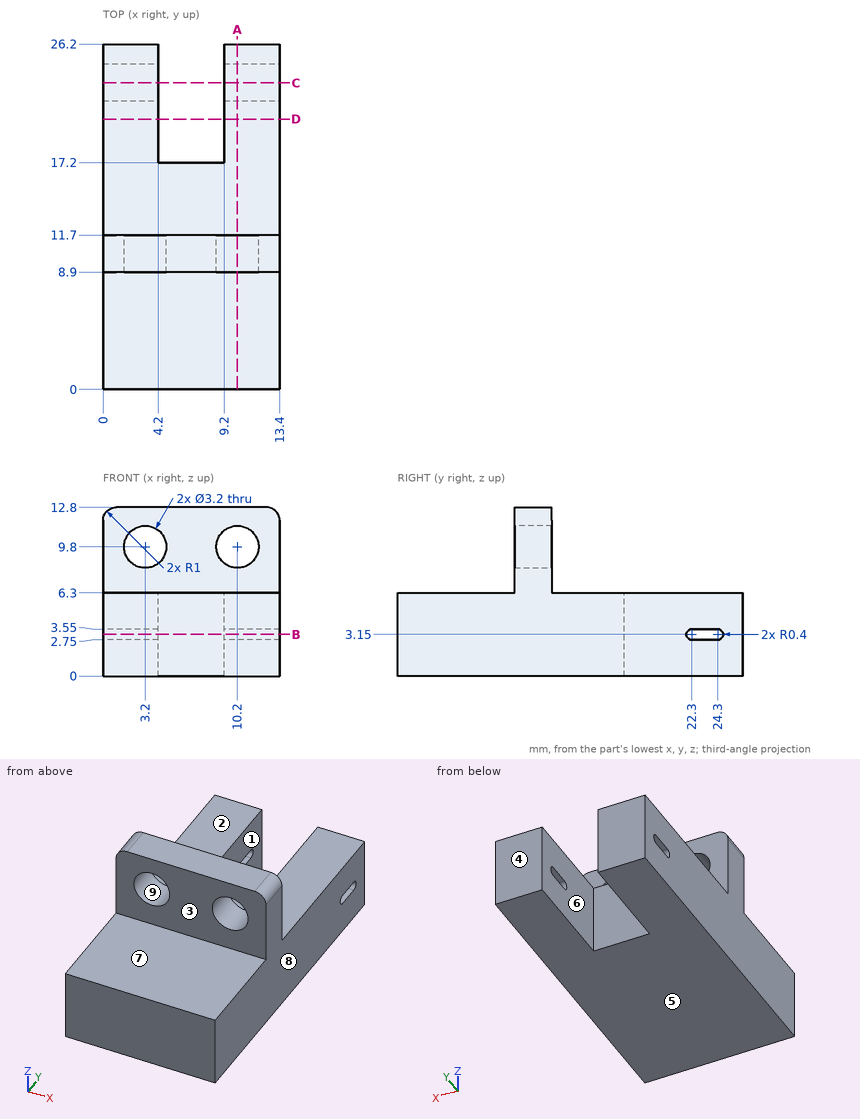
Job drawing, mm, ordinate dimensions from the low corner. One solid piece. A direction names the side the tool comes from. Give positions to 0.01 mm unless a question says otherwise; leave off trailing zeros. Write each loop counter-clockwise with the first axis right and the second up, starting at its lowest first coordinate (ties: lowest second). Pieces come first, ordered by that corner, then holes. Notation, with made-up numbers: M 15.5,47.25 L 47.5,47.25 A11 ccw 47.5,61.25 Z; hole C -11.75,70 d10. An arc over 180 degrees is marked long. Put each result on its own line as item: value. Start each with the question number.
(1) Band-saw the part on C-C, the plane y = 23.25. Write the cut outline in (x, z).
(2) Mould opens along X. For the marked faces 6, 7, 8 and 9 say: +X half, -X half, draft (parallel to the pull), parting line (faces both ways), or undercut.
(3) Which spindle directions (+Z, -Z, +X, -X, +Y, -Y) get a long thin tool onto all of the face, cutting with end or side? Do the marked faces 1, 2, 3, 4 and 5. Say none if no direction does.
(4) Flat gauge pins, fed straight in: pin 1 Ø7 at (x, z) = (5, 10) entering from +Y; pin 2 Ø1.5 at (x, z) = (6, 8) entering from -Y; pin 3 Ø0.6 at (x, y) = (1.5, 23.5) entering from +Z; pin 4 Ø1.9 at (x, z) = (3.2, 9.8) entering from +Y. Where does each tip first touch, or does it go through?
(5) Band-saw the part on A-A, the plane x = 10.2. Write the cut outline in (y, z).
(6) Band-saw the part on B-B, the plane z = 3.15. Write the cut outline in (x, y).
(7) Band-saw the part on D-D, the plane y = 20.5. Write the cut outline in (x, z), and give its area (3 significant figures).
(8) Probe L1, parallel to X at y = 11.1, z = 9.8; L2, parallel to Z at x = 12.5, y = 23.5; L3, parallel to Y at x = 8.25, z = 11.5. List the from-to ranges inside material, lowest first.
Response values:
1. outline: M 0,0 L 4.2,0 L 4.2,2.75 L 0,2.75 Z; M 0,3.55 L 4.2,3.55 L 4.2,6.3 L 0,6.3 Z; M 9.2,0 L 13.4,0 L 13.4,2.75 L 9.2,2.75 Z; M 9.2,3.55 L 13.4,3.55 L 13.4,6.3 L 9.2,6.3 Z
2. face 6: undercut
2. face 7: draft
2. face 8: +X half
2. face 9: undercut
3. face 1: +Z, -Z, +Y
3. face 2: +Z, +X, -X, +Y
3. face 3: +Z, +X, -X, -Y
3. face 4: +Z, -Z, +X, -X, +Y
3. face 5: -Z, +X, -X, +Y, -Y
4. pin 1: stops at y = 11.7
4. pin 2: stops at y = 8.9
4. pin 3: stops at z = 6.3
4. pin 4: passes through
5. outline: M 0,0 L 26.2,0 L 26.2,6.3 L 11.7,6.3 L 11.7,8.2 L 8.9,8.2 L 8.9,6.3 L 0,6.3 Z; M 8.9,11.4 L 11.7,11.4 L 11.7,12.8 L 8.9,12.8 Z; hole M 22.3,2.75 L 24.3,2.75 A0.4 ccw 24.3,3.55 L 22.3,3.55 A0.4 ccw Z
6. outline: M 0,0 L 13.4,0 L 13.4,21.9 L 9.2,21.9 L 9.2,17.2 L 4.2,17.2 L 4.2,21.9 L 0,21.9 Z; M 0,24.7 L 4.2,24.7 L 4.2,26.2 L 0,26.2 Z; M 9.2,24.7 L 13.4,24.7 L 13.4,26.2 L 9.2,26.2 Z
7. outline: M 0,0 L 4.2,0 L 4.2,6.3 L 0,6.3 Z; M 9.2,0 L 13.4,0 L 13.4,6.3 L 9.2,6.3 Z
7. area: 52.9 mm2
8. L1: x = 0 to 1.6, 4.8 to 8.6, 11.8 to 13.4
8. L2: z = 0 to 2.75, 3.55 to 6.3
8. L3: y = 8.9 to 11.7
